Can you work these out from the model? Positions are in its coordinate system, mm. Face numbers are marked on the shaded views. A direction names the side the tool comes from. Give positions to 0.01 mm unless a question says otherwise; leave off trailing zeros. Write each loop counter-clockwise with the first axis right and the second up, starting at its lowest first coordinate (ties: lowest second). Pieces come first, ordered by that corner, then holes. Notation, with made-up numbers: M 84.25,-12.75 L 90.25,-12.75 A16 cw 90.25,17.25 Z; hole C -12,13.5 d3. An arc over 180 degrees is marked long. Use CSV: the item, a comma, the result in double quotes. Start each with the question number.
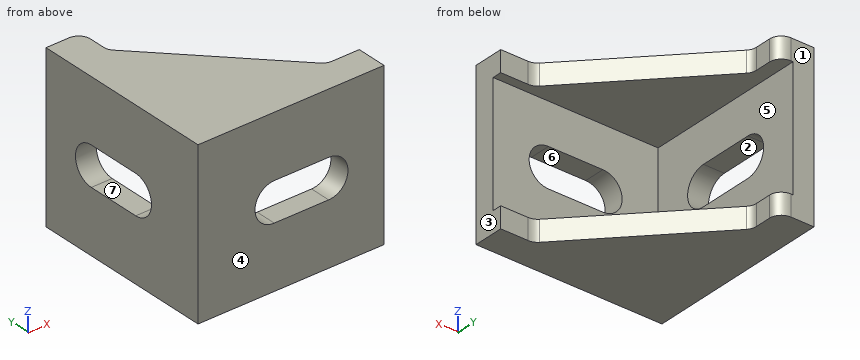
from build123d import *

# Parameters (mm, degrees)
BOSS_EXTRUDE1_DEPTH = 17.5
BOSS_EXTRUDE2_DEPTH = 4.5
CUT_EXTRUDE1_DEPTH  = 5.5
CUT_EXTRUDE2_DEPTH  = 5.5
FILLET1_R           = 2.54


with BuildPart() as part:
    # Sketch1 → Boss-Extrude1 (new body, symmetric)
    with BuildSketch(Plane.XY):
        Polygon((-20, 17.75), (-15.5, 17.75), (-15.5, -17.75), (20, -17.75), (20, -22.25), (-20, -22.25), align=None)
    extrude(amount=BOSS_EXTRUDE1_DEPTH, both=True)

    # Sketch2 → Boss-Extrude2 (add)
    with BuildSketch(Plane.XY.offset(17.5)):
        Polygon((-15.5, 17.75), (-12.5, 17.75), (-12.5, 10.75), (13, -15.75), (20, -15.75), (20, -17.75), (-15.5, -17.75), align=None)
    boss_extrude2 = extrude(amount=-BOSS_EXTRUDE2_DEPTH)

    # Mirror1: Boss-Extrude2 across plane
    add(boss_extrude2.mirror(Plane.XY))

    # Sketch3 → Cut-Extrude1 (cut, through all)
    with BuildSketch(Plane(origin=(-15.5, 0, 0), x_dir=(0, 0, -1), z_dir=(1, 0, 0))):
        with BuildLine():
            Line((4.15, 5.85), (4.15, -5.85))
            ThreePointArc((4.15, -5.85), (0, -10), (-4.15, -5.85))
            Line((-4.15, -5.85), (-4.15, 5.85))
            ThreePointArc((-4.15, 5.85), (0, 10), (4.15, 5.85))
        make_face()
    extrude(amount=-CUT_EXTRUDE1_DEPTH, mode=Mode.SUBTRACT)

    # Sketch4 → Cut-Extrude2 (cut, through all)
    with BuildSketch(Plane(origin=(0, -17.75, 0), x_dir=(1, 0, 0), z_dir=(0, 1, 0))):
        with BuildLine():
            Line((-3.6, 4.15), (8.1, 4.15))
            ThreePointArc((8.1, 4.15), (12.25, 0), (8.1, -4.15))
            Line((8.1, -4.15), (-3.6, -4.15))
            ThreePointArc((-3.6, -4.15), (-7.75, 0), (-3.6, 4.15))
        make_face()
    extrude(amount=-CUT_EXTRUDE2_DEPTH, mode=Mode.SUBTRACT)

    # Fillet1
    fillet1_edges = [part.edges().sort_by_distance(p)[0] for p in [
        (-12.5, 17.75, 15.25),
        (-12.5, 10.75, 15.25),
        (13, -15.75, 15.25),
        (13, -15.75, -15.25),
        (-12.5, 10.75, -15.25),
        (-12.5, 17.75, -15.25),
    ]]
    fillet(fillet1_edges, radius=FILLET1_R)


solid = part.part
(1) I want a section at C-C (x = -17). Write out the boundary of the cut face in (y, z), and give its area (3 significant figures).
(2) I want a section at A-A (z = 0). Write out the boundary of the cut face in (x, y), and give its area (3 significant figures).
(3) Please list where these lines run through material, in increasing order: L1, parallel to Z at x = -10, y = -16; L2, parallel to Z at x = -17, y = -0.5; L3, parallel to Y at x = 16.5, z = 9. Write a range as [from, to].
(4) I want a section at D-D (x = -5). Write out the boundary of the cut face in (y, z), and give its area (3 significant figures).
(5) Which directions (+Z, -Z, +X, -X, +Y, -Y) give clear straight access to the entire face, cutting with the end or side of a thin tool? Please do the marked faces 5, 6 and 7.
(6) Thinking about a two-plate mould opening in Y: for the marked faces 1, 2, 3 and 4, which applies, released by +Y, released by -Y, zero draft, split by the parting line, or undercut?
(7) Will these pins go through, and if not, where does the flat tip stop? pin 1 Ø3 at (x, z) = (1, 10.5) entering from +Y; pin 2 Ø1.7 at (y, z) = (14.5, 15.5) entering from +X; pin 3 Ø2 at (x, z) = (18.5, -15.5) entering from +Y.
(8) I want a section at B-B (y = -18.5). Write out the boundary of the cut face in (x, z), and give its area (3 significant figures).
Geometry results:
1,outline,"M -22.25,-17.5 L 17.75,-17.5 L 17.75,17.5 L -22.25,17.5 Z; hole M -5.85,-4.15 L 5.85,-4.15 A4.15 ccw 5.85,4.15 L -5.85,4.15 A4.15 ccw Z"
1,area,"1,250 mm2"
2,outline,"M -20,-22.25 L -7.75,-22.25 L -7.75,-17.75 L -15.5,-17.75 L -15.5,-10 L -20,-10 Z; M -20,10 L -15.5,10 L -15.5,17.75 L -20,17.75 Z; M 12.25,-22.25 L 20,-22.25 L 20,-17.75 L 12.25,-17.75 Z"
2,area,"160 mm2"
3,L1,"z = [-17.5, -13], [13, 17.5]"
3,L2,"z = [-17.5, -4.15], [4.15, 17.5]"
3,L3,"y = [-22.25, -17.75]"
4,outline,"M -22.25,-17.5 L 2.96,-17.5 L 2.96,-13 L -17.75,-13 L -17.75,-3.91 L -22.25,-3.91 Z; M -22.25,3.91 L -17.75,3.91 L -17.75,13 L 2.96,13 L 2.96,17.5 L -22.25,17.5 Z"
4,area,"309 mm2"
5,face 5,"+X, +Y"
5,face 6,"+Y, -Y"
5,face 7,"+X, -X"
6,face 1,"released by +Y"
6,face 2,"undercut"
6,face 3,"zero draft"
6,face 4,"released by -Y"
7,pin 1,"stops at y = -17.75"
7,pin 2,"stops at x = -12.5"
7,pin 3,"stops at y = -15.75"
8,outline,"M -20,-17.5 L 20,-17.5 L 20,17.5 L -20,17.5 Z; hole M -3.6,-4.15 L 8.1,-4.15 A4.15 ccw 8.1,4.15 L -3.6,4.15 A4.15 ccw Z"
8,area,"1,250 mm2"
